from build123d import *

# Parameters (mm, degrees)
F2_R = 4.99999


# Not quite as in the source:
# - a fillet or chamfer is up to 0.001 mm smaller than in the source, because OpenCascade refuses the exact size


with BuildPart() as f1:
    # F0 (on Front) → F1 (revolve)
    with BuildSketch(Plane.XZ):
        Polygon((-20, 11.6256596521), (0, 11.6256596521), (20, 11.6256596521), (20, 26.6256596521), (15, 26.6256596521), (15, 30), (30, 30), (30, 50), (0, 50), (-30, 50), (-30, 30), (-15, 30), (-15, 26.6256596521), (-20, 26.6256596521), align=None)
    revolve(axis=Axis((30.7941585779, 0, 0), (1, 0, 0)))

    # F2 (radius 5 in the source; OpenCascade refuses exactly that, so slightly less here)
    f2_edges = [f1.edges().sort_by_distance(p)[0] for p in [
        (20, 0, -11.62566),
        (20, 0, -26.62566),
    ]]
    fillet(f2_edges, radius=F2_R)


solid = f1.part
Build history of the part. All positions in model axes, mm. A direction names the side the tool comes from. Round coordinates to 2 decimals unless told otherwise and drop trailing zeros. Write each loop counter-clockwise with the first axis right and the second up, starting at its lowest first coordinate (ties: lowest second). Pieces come first, ordered by that corner, then holes. Notation, with made-up numbers: M 39.5,-36 L 54.5,-36 A14 ccw 54.5,-12 Z; hole C 84,-33.75 d1. An arc over 180 degrees is marked long. Answer as a JSON object with one key per item and string values. Group by question number.
(1) Flat gauge pins, fed straight in: pin 1 (12 mm diameter, centred on x = -15.5, y = -20, fed in from +Z); pin 2 (10 mm diameter, centred on x = -8, z = -28, fed in from -Y); pin 3 (16 mm diameter, centred on y = 9, z = 2.5, fed in from -X); pin 4 (18.5 mm diameter, centred on y = 0, z = 0, fed in from -X). Where does each tip first touch, or does it go through?
(2) Cut at D-D (x = 13). Give the cut face in (y, z).
(3) Cut at C-C (y = 28). Give the cut face in (x, z).
(4) Mould opens along Z. For faces 4 (the cylindrical face through (-0.42, -15.02, 47.69)), 5 (the flat face through (30, 22, -22)), 6 (the cylindrical face through (22.6, -1.32, -29.97)) say: pulls with the +Z half, pulls with the -Z half, needs draft (parallel to the pull), parting line crosses it, or undercut.
(5) Which spindle directions (+Z, -Z, +X, -X, +Y, -Y) get a long thin tool onto all of the face, cutting with end or side? Do faces 1 (the flat face through (-30, 22, 22)), 2 (the flat face through (-20, 6, 11)), 3 (the flat face through (15, 24.3, 11.3)). Say none if no direction does.
(6) Drill centre lines: L1, parallel to Z at x = -18.75, y = 0; L2, parallel to Y at x = -27, z = 0. Where is each one in solid material? Low to high.
Responses:
{
 "1": {"pin 1": "stops at z = 48", "pin 2": "stops at y = -44.4", "pin 3": "stops at x = -20", "pin 4": "passes through"},
 "2": {"outline": "C 0,0 d100; hole C 0,0 d23.25"},
 "3": {"outline": "M -30,-41.42 L 30,-41.42 L 30,-10.77 L 15,-10.77 L 15,10.77 L 30,10.77 L 30,41.42 L -30,41.42 L -30,10.77 L -15,10.77 L -15,-10.77 L -30,-10.77 Z"},
 "4": {"face 4": "parting line crosses it", "face 5": "needs draft", "face 6": "undercut"},
 "5": {"face 1": "+Z, -Z, -X, +Y, -Y", "face 2": "-X", "face 3": "+X"},
 "6": {"L1": "z = -50 to -30, -26.63 to -11.63, 11.63 to 26.63, 30 to 50", "L2": "y = -50 to -30, 30 to 50"}
}
